from build123d import *

# Parameters (mm, degrees)
EXTRUDE_1_DEPTH        = 50
HOLE_WIZARD_M4_1_D     = 3.3
HOLE_WIZARD_M4_1_DEPTH = 10.1
HOLE_WIZARD_M4_1_TIP   = 0.991420021
SKETCH_2_R             = 10.1
CUT_EXTRUDE_1_DEPTH    = 50
HOLE_WIZARD_M4_2_D     = 3.3


with BuildPart() as part:
    # 草图1 → 凸台-拉伸1 (new body)
    with BuildSketch(Plane(origin=(0, 0, 0), x_dir=(1, 0, 0), z_dir=(0, 1, 0))):
        Polygon((-12.088519272, -36.909676467), (17.911480728, 15.05184776), (32.903920346, 14.575660494), (2.903920346, -37.385863733), align=None)
    extrude(amount=EXTRUDE_1_DEPTH)

    # M4 螺纹孔1
    with Locations(Plane(origin=(10.045844782, 0, 25.015687746), x_dir=(-0.5, 0, 0.866025404), z_dir=(0.866025404, 0, 0.5))):
        with Locations((-17.783614548, -17.5), (-4.793233491, -40), (8.197147566, -17.5)):
            Hole(HOLE_WIZARD_M4_1_D / 2, depth=HOLE_WIZARD_M4_1_DEPTH)
            with Locations((0, 0, -(HOLE_WIZARD_M4_1_DEPTH + HOLE_WIZARD_M4_1_TIP / 2))):  # 118° drill point
                Cone(0, HOLE_WIZARD_M4_1_D / 2, HOLE_WIZARD_M4_1_TIP, mode=Mode.SUBTRACT)

    # 草图2 → 切除-拉伸1 (cut)
    with BuildSketch(Plane(origin=(-1.404680066, 0, 18.404724143), x_dir=(-0.5, 0, 0.866025404), z_dir=(-0.866025404, 0, -0.5))):
        with Locations((-4.793233491, 25)):
            Circle(SKETCH_2_R)
    extrude(amount=-CUT_EXTRUDE_1_DEPTH, mode=Mode.SUBTRACT)

    # M4 螺纹孔2 (through all)
    with Locations(Plane(origin=(0.495643511, 0, -15.60500656), x_dir=(-0.999495975, 0, -0.031745818), z_dir=(0.031745818, 0, -0.999495975))):
        with Locations((-24.92461967, 35), (-24.92461967, 15)):
            Hole(HOLE_WIZARD_M4_2_D / 2)


solid = part.part
Work out the finished part from the listing and answer in its coordinate system (mm). A direction names the side the tool comes from. Round coordinates to 2 decimals unless told otherwise and drop trailing zeros. Order: outer loops, then holes, each group sorted by start corner. A loop starts at its lowest first (then second) coordinate and runs counter-clockwise, first axis right, second up. Notation, with made-up numbers: M 87.5,3.5 L 141.5,3.5 A21 cw 141.5,35.5 Z; hole C 4,21 d4. An arc over 180 degrees is marked long. One line per item, written item: value.
Q1. Find section D-D on y = 9. Write down the section's boundary in (x, z), then the cut area to 3 significant figures.
Derived:
outline: M -12.09,36.91 L 17.91,-15.05 L 32.9,-14.58 L 2.9,37.39 Z
area: 793 mm²
Q2. Find section B-B on y = 23. Write down the section's boundary in (x, z).
Derived:
outline: M -12.09,36.91 L -3.96,22.83 L 7.49,29.44 L 2.9,37.39 Z; M 5.94,5.68 L 17.91,-15.05 L 32.9,-14.58 L 17.39,12.29 Z
Q3. Determine the mould class of faces 1 (the face through (12, 50, 11)), 2 (the face through (14.396, 15.864, 7.24)), 3 (the face through (6.035, 19.094, 5.519)), 4 (the face through (-3.586, 17.258, 26.788)) for opening direction Y: released by +Y, released by -Y, zero draft, split by the parting line, or undercut.
Derived:
face 1: released by +Y
face 2: undercut
face 3: zero draft
face 4: undercut
Q4. Flat-ended cylindrical pins translate along their axes: pin 1 (2 mm diameter, centred on x = -1.5, y = 38.5, fed in from -Z); pin 2 (5 mm diameter, centred on y = 14.5, z = 18.5, fed in from +X); pin 3 (10 mm diameter, centred on y = 20, z = -5.5, fed in from -X). Find the tip coordinate at first contact, or state that the pin passes through.
Derived:
pin 1: z = 16.84
pin 2: x = 15.25
pin 3: x = 9.51
Q5. Find section A-A on y = 29. Write down the section's boundary in (x, z), then the cut area to 3 significant figures.
Derived:
outline: M -12.09,36.91 L -3.65,22.29 L 7.81,28.9 L 2.9,37.39 Z; M 5.63,6.22 L 17.91,-15.05 L 32.9,-14.58 L 17.08,12.83 Z
area: 548 mm²
Q6. Straight lines are drawn through the part: line 1 (Y direction, x = 3, z = 14.5); line 2 (Z direction, x = 3.5, y = 34); line 3 (Z direction, x = -9, y = 7). For each, find the intervals that lie inside material, in ascending order.
Derived:
line 1: 0 to 14.93, 35.07 to 50
line 2: 9.91 to 10.41, 20.99 to 36.35
line 3: 31.56 to 37.01
Q7. Find section C-C on x = 28. Write down the section's boundary in (y, z), then the cut area to 3 significant figures.
Derived:
outline: M 0,-14.73 L 50,-14.73 L 50,-6.08 L 0,-6.08 Z
area: 432 mm²
Q8. For faces 5 (the face through (9.404, 17.258, 4.288)), 6 (the face through (12, 0, 11)), determine the directions among +Z, -Z, +X, -X, +Y, -Y from which every point of the face is accessible in a straight line to the end or side of a thin tool.
Derived:
face 5: none
face 6: +Z, -Z, +X, -X, -Y
